```python
from build123d import *

# Parameters (mm, degrees)
SKETCH1_R         = 17.78
EXTRUDE1_DEPTH    = 2.54
CIRPATTERN2_COUNT = 8
SKETCH7_R         = 3.175
EXTRUDE2_DEPTH    = 2.54


with BuildPart() as part:
    # Sketch1 → Extrude1 (new body)
    with BuildSketch(Plane.XY):
        Circle(SKETCH1_R)
    extrude(amount=EXTRUDE1_DEPTH)

    # Sketch6 → #39 (0.0995) Diameter Hole2 (revolve, cut)
    with BuildSketch(Plane(origin=(0, 15.24, 2.54), x_dir=(0, -1, 0), z_dir=(1, 0, 0))):
        Polygon((0, 0), (0, 10.919277521), (1.26365, 10.16), (1.26365, 0), align=None)
    f_39_0_0995_diameter_hole2 = revolve(axis=Axis((0, 15.24, 8.89), (0, 0, -1)), mode=Mode.SUBTRACT)

    # CirPattern2: #39 (0.0995) Diameter Hole2 ×8 about axis
    cirpattern2_axis = Axis((0, 0, 0), (0, 0, 1))
    for i in range(1, CIRPATTERN2_COUNT):
        add(f_39_0_0995_diameter_hole2.rotate(cirpattern2_axis, i * 360 / CIRPATTERN2_COUNT), mode=Mode.SUBTRACT)

    # Sketch7 → Extrude2 (add)
    with BuildSketch(Plane(origin=(0, 0, 0), x_dir=(-1, 0, 0), z_dir=(0, 0, -1))):
        Circle(SKETCH7_R)
    extrude(amount=EXTRUDE2_DEPTH)


solid = part.part
```
Geometry check sheet. Reference: the model listing, model coordinates, mm. Coordinates: 2 decimals unless noted, no trailing zeros. Order: outer loops, then holes, each group sorted by start corner. A loop starts at its lowest first (then second) coordinate and runs counter-clockwise, first axis right, second up. Notation, with made-up numbers: (85, 31) - (118, 31) arc R11 cw to (118, 48) - close; hole circle Ø1 at (9.5, 20). An arc over 180 degrees is marked (long way). Use one line per item in the form item = value.
1. Section check A-A (y = 0). Record the boundary of the cut face in (x, z) (3 decimals).
Here are the results:
outline = (-17.78, 0) - (-16.504, 0) - (-16.504, 2.54) - (-17.78, 2.54) - close; (-13.976, 0) - (-3.175, 0) - (-3.175, -2.54) - (3.175, -2.54) - (3.175, 0) - (13.976, 0) - (13.976, 2.54) - (-13.976, 2.54) - close; (16.504, 0) - (17.78, 0) - (17.78, 2.54) - (16.504, 2.54) - close
2. Section check D-D (z = 0.6). State how many separate pieces and enclosed holes the cut face has, then the cut area to 3 significant figures.
Here are the results:
separate_pieces = 1
enclosed_holes = 8
area = 953 mm²
3. Draft check along Y on faces 1 (the face through (10.098, -11.842, 1.288)), 2 (the face through (0, -4, 0)), 3 (the face through (0.69, -3.1, -1.25)). Enter one of: pulls with the +Y half, pulls with the -Y half, needs draft (parallel to the pull), parting line crosses it, or undercut.
Here are the results:
face_1 = undercut
face_2 = needs draft
face_3 = parting line crosses it
4. Section check C-C (y = 15). Record the boundary of the cut face in (x, z).
Here are the results:
outline = (-9.55, 0) - (-1.24, 0) - (-1.24, 2.54) - (-9.55, 2.54) - close; (1.24, 0) - (9.55, 0) - (9.55, 2.54) - (1.24, 2.54) - close
5. Scan lines: line 1 (X direction, y = 0.5, z = 2.2); line 2 (Z direction, x = -0.5, y = -10); line 3 (X direction, y = -15.24, z = 0.95). Record each from-to range of solid material in increasing order.
Here are the results:
line_1 = -17.77 to -16.4, -14.08 to 14.08, 16.4 to 17.77
line_2 = 0 to 2.54
line_3 = -9.16 to -1.26, 1.26 to 9.16
6. Gauge pin test, flat ends, axial feed: pin 1 (1.5 mm diameter, centred on y = 7, z = -0.5, fed in from +X); pin 2 (2 mm diameter, centred on x = 0, y = 15.24, fed in from +Z); pin 3 (3 mm diameter, centred on x = 11.5, z = -1, fed in from -Y); pin 4 (1.5 mm diameter, centred on x = -12.5, z = 0.5, fed in from -Y). Record the tip position at first contact, or that the pin passes through.
Here are the results:
pin_1 = 16.57
pin_2 = through
pin_3 = -14.43
pin_4 = -13.34
